Build history of the part. All positions in model axes, mm. Face numbers are marked on the shaded views. A direction names the side the tool comes from. Coordinates: 2 decimals unless noted, no trailing zeros. Write each loop counter-clockwise with the first axis right and the second up, starting at its lowest first coordinate (ties: lowest second). Pieces come first, ordered by that corner, then holes.
```python
from build123d import *

# Parameters (mm, degrees)
ESQUISSE1_W             = 30
ESQUISSE1_H             = 28
BOSS_EXTRU_1_DEPTH      = 8
ENL_V_MAT_EXTRU_1_DEPTH = 9
ENL_V_MAT_EXTRU_2_DEPTH = 4.2
CHANFREIN1_SIZE         = 18
CHANFREIN1_SIZE2        = 6.551464217
CHANFREIN1_PART_2_SIZE  = 18
CHANFREIN1_PART_2_SIZE2 = 6.551464217
CONG_1_R                = 2
ESQUISSE4_W             = 2.6
ESQUISSE4_H             = 6.2
ENL_V_MAT_EXTRU_3_DEPTH = 9
ESQUISSE5_R             = 1.7
ENL_V_MAT_EXTRU_4_DEPTH = 16
ESQUISSE6_W             = 6
ESQUISSE6_H             = 5.5
ESQUISSE6_R             = 1.7
BOSS_EXTRU_2_DEPTH      = 1.6
CONG_2_R                = 1


with BuildPart() as part:
    # Esquisse1 → Boss.-Extru.1 (new body)
    with BuildSketch(Plane.XY):
        with Locations((7, 0)):
            Rectangle(ESQUISSE1_W, ESQUISSE1_H)
    extrude(amount=BOSS_EXTRU_1_DEPTH)

    # Esquisse2 → Enlèv. mat.-Extru.1 (cut, through all)
    with BuildSketch(Plane.XY.offset(8)):
        with BuildLine():
            Line((-3, 2.2), (7, 2.2))
            ThreePointArc((7, 2.2), (9.2, 0), (7, -2.2))
            Line((7, -2.2), (-3, -2.2))
            ThreePointArc((-3, -2.2), (-5.2, 0), (-3, 2.2))
        make_face()
    extrude(amount=-ENL_V_MAT_EXTRU_1_DEPTH, mode=Mode.SUBTRACT)

    # Esquisse3 → Enlèv. mat.-Extru.2 (cut)
    with BuildSketch(Plane.XY.offset(8)):
        with BuildLine():
            Line((-3, 4), (7, 4))
            ThreePointArc((7, 4), (11, 0), (7, -4))
            Line((7, -4), (-3, -4))
            ThreePointArc((-3, -4), (-7, 0), (-3, 4))
        make_face()
    extrude(amount=-ENL_V_MAT_EXTRU_2_DEPTH, mode=Mode.SUBTRACT)

    # Chanfrein1
    chanfrein1_edges = [part.edges().sort_by_distance(p)[0] for p in [
        (-8, 14, 4),
    ]]
    chanfrein1_side = [part.faces().sort_by_distance(p)[0] for p in [
        (7, 14, 4),
    ]]
    chamfer(chanfrein1_edges, length=CHANFREIN1_SIZE, length2=CHANFREIN1_SIZE2, reference=chanfrein1_side[0])

    # Chanfrein1 part 2
    chanfrein1_part_2_edges = [part.edges().sort_by_distance(p)[0] for p in [
        (-8, -14, 4),
    ]]
    chanfrein1_part_2_side = [part.faces().sort_by_distance(p)[0] for p in [
        (7, -14, 4),
    ]]
    chamfer(chanfrein1_part_2_edges, length=CHANFREIN1_PART_2_SIZE, length2=CHANFREIN1_PART_2_SIZE2, reference=chanfrein1_part_2_side[0])

    # Congé1
    cong_1_edges = [part.edges().sort_by_distance(p)[0] for p in [
        (10, -14, 4),
        (-8, 7.448535783, 4),
        (-8, -7.448535783, 4),
        (10, 14, 4),
    ]]
    fillet(cong_1_edges, radius=CONG_1_R)

    # Esquisse4 → Enlèv. mat.-Extru.3 (cut, through all)
    with BuildSketch(Plane(origin=(0, 0, 0), x_dir=(-1, 0, 0), z_dir=(0, 0, -1))):
        with Locations((-17.7, -9.35)):
            Rectangle(ESQUISSE4_W, ESQUISSE4_H)
        with Locations((-17.7, 9.35)):
            Rectangle(ESQUISSE4_W, ESQUISSE4_H)
    extrude(amount=-ENL_V_MAT_EXTRU_3_DEPTH, mode=Mode.SUBTRACT)

    # Esquisse5 → Enlèv. mat.-Extru.4 (cut)
    with BuildSketch(Plane(origin=(22, 0, 0), x_dir=(0, 0, -1), z_dir=(1, 0, 0))):
        with Locations((-3, 9.25)):
            Circle(ESQUISSE5_R)
        with Locations((-3, -9.25)):
            Circle(ESQUISSE5_R)
    extrude(amount=-ENL_V_MAT_EXTRU_4_DEPTH, mode=Mode.SUBTRACT)

    # Esquisse6 → Boss.-Extru.2 (add)
    with BuildSketch(Plane(origin=(22, 0, 0), x_dir=(0, 0, -1), z_dir=(1, 0, 0))):
        with Locations((-3, -9.25)):
            Rectangle(ESQUISSE6_W, ESQUISSE6_H)
        with Locations((-3, -9.25)):
            Circle(ESQUISSE6_R, mode=Mode.SUBTRACT)
        with Locations((-3, 9.25)):
            Rectangle(ESQUISSE6_W, ESQUISSE6_H)
        with Locations((-3, 9.25)):
            Circle(ESQUISSE6_R, mode=Mode.SUBTRACT)
    extrude(amount=BOSS_EXTRU_2_DEPTH)

    # Congé2
    cong_2_edges = [part.edges().sort_by_distance(p)[0] for p in [
        (22, -12, 3),
        (22, 6.5, 3),
        (22, -9.25, 6),
        (22, -6.5, 3),
        (22, 9.25, 6),
        (22, 12, 3),
    ]]
    fillet(cong_2_edges, radius=CONG_2_R)


solid = part.part
```
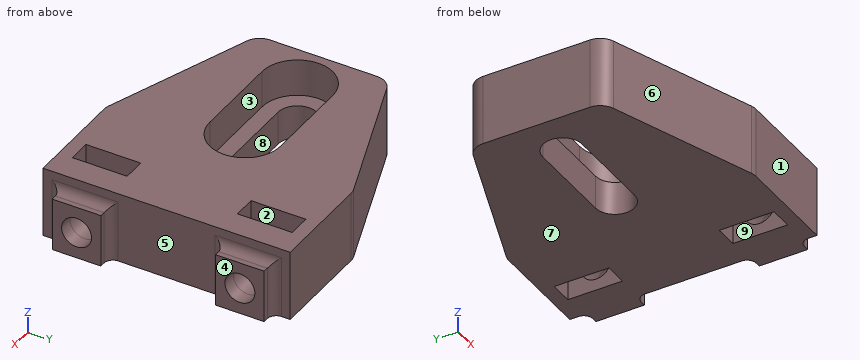
1. Probe line 1 along Y through (x, z) = (18.5, 7.75); line 2 along Y through (x, z) = (20.55, 3); line 3 along Y through (x, z) = (23.1, 3). List the from-to ranges inside material, lowest first.
Computed values:
line 1: y = -14 to -12.45, -6.25 to 6.25, 12.45 to 14
line 2: y = -14 to -10.95, -7.55 to 7.55, 10.95 to 14
line 3: y = -12 to -10.95, -7.55 to -6.5, 6.5 to 7.55, 10.95 to 12
2. Flat gauge pins, fed straight in: pin 1 (1.3 mm diameter, centred on x = 3.5, z = 6, fed in from +Y); pin 2 (0.5 mm diameter, centred on x = 23.5, y = 9.5, fed in from +Z); pin 3 (3 mm diameter, centred on x = 16.5, y = 10.5, fed in from -Z); pin 4 (2.5 mm diameter, centred on y = -9.25, z = 3, fed in from +X). Where does each tip first touch, or does it go through?
Computed values:
pin 1: stops at y = 11.87
pin 2: stops at z = 6
pin 3: stops at z = 0
pin 4: stops at x = 6
3. Saw through at A-A on y = 0. List the corners of the cut face in (x, z), plus the area to 3 significant figures.
Computed values:
outline: (-8, 0) - (-5.2, 0) - (-5.2, 3.8) - (-7, 3.8) - (-7, 8) - (-8, 8) - close; (9.2, 0) - (22, 0) - (22, 8) - (11, 8) - (11, 3.8) - (9.2, 3.8) - close
area: 110 mm2
4. Saw through at C-C on x = 21.5. List the corners of the cut face in (y, z).
Computed values:
outline: (-14, 0) - (14, 0) - (14, 8) - (-14, 8) - close; hole circle Ø3.4 at (-9.25, 3); hole circle Ø3.4 at (9.25, 3)
5. Saw through at B-B on x = 8. List the corners of the cut face in (y, z).
Computed values:
outline: (-13.27, 0) - (-1.96, 0) - (-1.96, 3.8) - (-3.87, 3.8) - (-3.87, 8) - (-13.27, 8) - close; (1.96, 0) - (13.27, 0) - (13.27, 8) - (3.87, 8) - (3.87, 3.8) - (1.96, 3.8) - close; hole circle Ø3.4 at (-9.25, 3); hole circle Ø3.4 at (9.25, 3)
6. Mould opens along X. For the marked faces 6, 7, 8 and 9 say: +X half, -X half, draft (parallel to the pull), parting line (faces both ways), or undercut.
Computed values:
face 6: -X half
face 7: draft
face 8: undercut
face 9: undercut
7. Saw through at D-D on y = 9.25. List the corners of the cut face in (x, z).
Computed values:
outline: (-3.05, 0) - (16.4, 0) - (16.4, 1.3) - (6, 1.3) - (6, 4.7) - (16.4, 4.7) - (16.4, 8) - (-3.05, 8) - close; (19, 0) - (23.6, 0) - (23.6, 1.3) - (19, 1.3) - close; (19, 4.7) - (23.6, 4.7) - (23.6, 6) - (23, 6) arc R1 cw to (22, 7) - (22, 8) - (19, 8) - close
8. 3-axis set-ups, long thin cutter, end or side, ignore diameter. For the marked faces 1, 2, 3, 4 and 5: which of +Z, -Z, +X, -X, +Y, -Y reach the whole face in a straight line?
Computed values:
face 1: +Z, -Z, +X, -X, -Y
face 2: +Z, -Z
face 3: +Z
face 4: +Z, -Z, +X, +Y, -Y
face 5: +Z, +X
